Job drawing, mm, ordinate dimensions from the low corner. One solid piece. A direction names the side the tool comes from. Coordinates: 2 decimals unless noted, no trailing zeros. Write each loop counter-clockwise with the first axis right and the second up, starting at its lowest first coordinate (ties: lowest second). Pieces come first, ordered by that corner, then holes. Notation, with made-up numbers: (25, 86.5) - (58, 86.5) arc R22 cw to (58, 119.5) - close; hole circle Ø2 at (-40, 79.25). An arc over 180 degrees is marked (long way). Use a Markdown table: item, result.
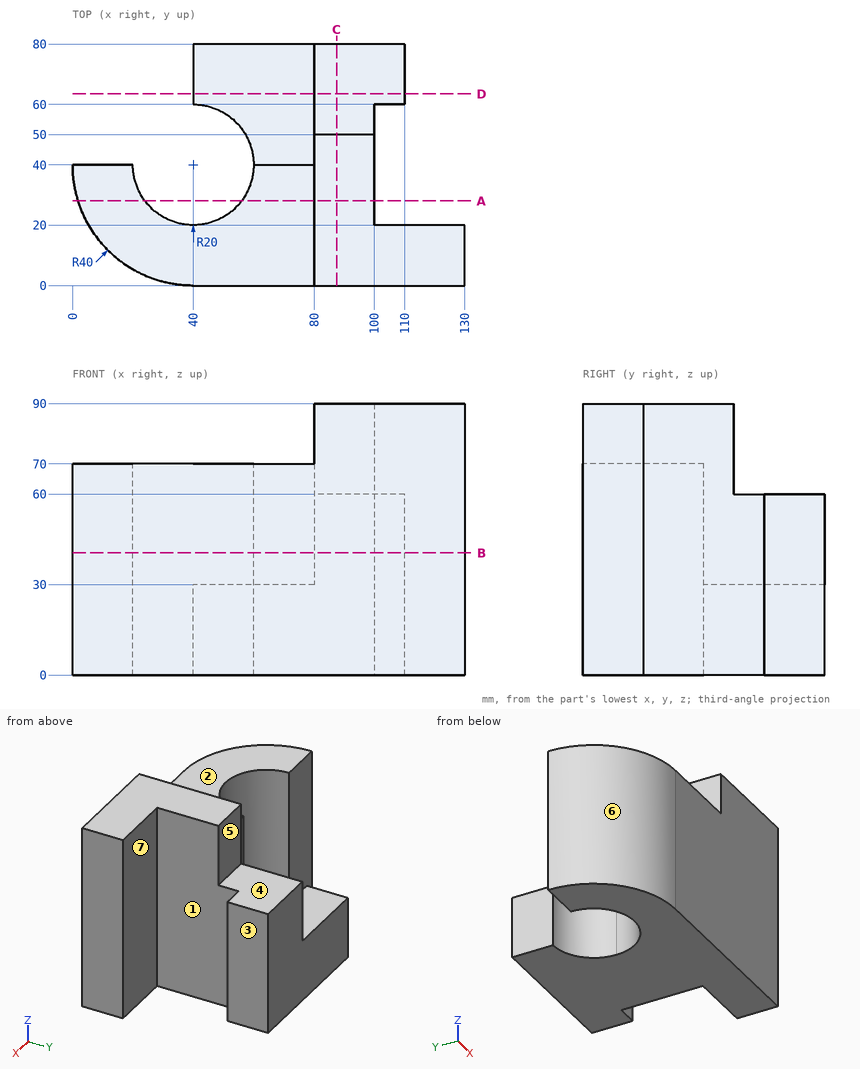
Item 1: Drill centre lines: probe 1 along X at (y, z) = (24.5, 86.5); probe 2 along Z at (x, y) = (61.5, 27.5); probe 3 along Y at (x, z) = (113, 40.5). Where is each one in solid material? Low to high.
From the geometry:
| item | result |
|---|---|
| probe 1 | 80 to 100 |
| probe 2 | 0 to 70 |
| probe 3 | 0 to 20 |
Item 2: Two-plate mould, pull along Y, no slides. Class the marked faces 4, 5, 6 and 7: pulls with the +Y half, pulls with the -Y half, needs draft (parallel to the pull), parting line crosses it, or undercut.
From the geometry:
| item | result |
|---|---|
| face 4 | needs draft |
| face 5 | pulls with the +Y half |
| face 6 | pulls with the -Y half |
| face 7 | undercut |
Item 3: Band-saw the part on B-B, the plane z = 40.5. Give the cut face in (x, y), then the cut area to 3 significant figures.
From the geometry:
| item | result |
|---|---|
| outline | (0, 40) arc R40 ccw to (40, 0) - (130, 0) - (130, 20) - (100, 20) - (100, 60) - (110, 60) - (110, 80) - (80, 80) - (80, 40) - (60, 40) arc R20 cw to (20, 40) - close |
| area | 4,630 mm^2 |
Item 4: Which spindle directions (+Z, -Z, +X, -X, +Y, -Y) get a long thin tool onto all of the face, cutting with end or side? Do the marked faces 1, 2 and 3. Say none if no direction does.
From the geometry:
| item | result |
|---|---|
| face 1 | +Z, -Z, +X |
| face 2 | +Z, -X, +Y, -Y |
| face 3 | +Z, -Z, +X, +Y |
Item 5: Band-saw the part on A-A, the plane y = 28. Give the cut face in (x, z), then the cut area to 3 significant figures.
From the geometry:
| item | result |
|---|---|
| outline | (1.84, 0) - (24, 0) - (24, 70) - (1.84, 70) - close; (56, 0) - (100, 0) - (100, 90) - (80, 90) - (80, 70) - (56, 70) - close |
| area | 5,030 mm^2 |
Item 6: Band-saw the part on C-C, the plane x = 87.5. Give the cut face in (y, z).
From the geometry:
| item | result |
|---|---|
| outline | (0, 0) - (80, 0) - (80, 60) - (50, 60) - (50, 90) - (0, 90) - close |
Item 7: Band-saw the part on D-D, the plane y = 63.5. Give the cut face in (x, z), then the cut area to 3 significant figures.
From the geometry:
| item | result |
|---|---|
| outline | (40, 0) - (110, 0) - (110, 60) - (80, 60) - (80, 30) - (40, 30) - close |
| area | 3,000 mm^2 |
Item 8: Drop flat-ended pins along their axis: P1, Ø16, axis at x = 71, z = 52, coming from the +Y side; P2, Ø12, axis at y = 11, z = 31, coming from the -X side; P3, Ø10, axis at x = 53, y = 69.5, coming from the +Z side. Give the stop position or say it passes through.
From the geometry:
| item | result |
|---|---|
| P1 | y = 40 |
| P2 | x = 7.27 |
| P3 | z = 30 |
